```python
from build123d import *

# Parameters (mm, degrees)
SKETCH_1_R          = 2
EXTRUDE_1_DEPTH     = 5
SKETCH_2_R          = 0.35
SKETCH_5_R          = 2.75
SKETCH_5_R_2        = 1.75
CUT_EXTRUDE_1_DEPTH = 4


with BuildPart() as part:
    # Эскиз1 → Бобышка-Вытянуть1 (new body)
    with BuildSketch(Plane(origin=(0, 0, 0), x_dir=(0, 0, -1), z_dir=(1, 0, 0))):
        Circle(SKETCH_1_R)
    extrude_1 = extrude(amount=EXTRUDE_1_DEPTH)

    # По траектории1: sweep along a path in Эскиз3
    with BuildLine(Plane.XY) as sweep_1_path:
        Line((5, 0), (9.16, 0))
        ThreePointArc((9.16, 0), (9.867106781, -0.292893219), (10.16, -1))
        Line((10.16, -1), (10.16, -8))
    # Эскиз2 → По траектории1 (sweep)
    with BuildSketch(Plane(origin=(5, 0, 0), x_dir=(0, 0, -1), z_dir=(1, 0, 0))):
        Circle(SKETCH_2_R)
    sweep_1 = sweep(path=sweep_1_path.line)

    # Зеркальное отражение1: Бобышка-Вытянуть1, По траектории1 across Right Plane
    add(extrude_1.mirror(Plane(origin=(0, 0, 0), x_dir=(0, 0, -1), z_dir=(1, 0, 0))))
    add(sweep_1.mirror(Plane(origin=(0, 0, 0), x_dir=(0, 0, -1), z_dir=(1, 0, 0))))

    # Эскиз5 → Вырез-Вытянуть-Тонкостенный1 (cut, symmetric)
    with BuildSketch(Plane(origin=(0, 0, 0), x_dir=(0, 0, -1), z_dir=(1, 0, 0))):
        Circle(SKETCH_5_R)
        Circle(SKETCH_5_R_2, mode=Mode.SUBTRACT)
    extrude(amount=CUT_EXTRUDE_1_DEPTH, both=True, mode=Mode.SUBTRACT)


solid = part.part
```
Verification items for the finished model (mm, model axes). Round coordinates to 2 decimals unless told otherwise and drop trailing zeros. Write each loop counter-clockwise with the first axis right and the second up, starting at its lowest first coordinate (ties: lowest second). Pieces come first, ordered by that corner, then holes. Notation, with made-up numbers: (68.5, 87) - (92.5, 87) arc R27 cw to (92.5, 124) - close; hole circle Ø8 at (9, 11.25). An arc over 180 degrees is marked (long way). Answer as a JSON object with one key per item and string values. Group by question number.
Q1. Thickness scan on line 1 (X direction, y = 1.75, z = 0.65); line 2 (X direction, y = 0.5, z = -1.6); line 3 (Y direction, x = -0.5, z = -0.1). Record the ranges inside material, lowest first.
Q2. Section check C-C, the plane x = 6. Enter the section's corners in (y, z), plus the area to 3 significant figures.
Q3. Section check B-B, the plane y = -7. Enter the section's corners in (x, z), plus the area to 3 significant figures.
Q4. Go/stop test with flat-tipped pins: pin 1 Ø1.2 at (y, z) = (1, 0.5) entering from -X; pin 2 Ø1.5 at (x, z) = (8, 0.5) entering from +Y; pin 3 Ø2 at (y, z) = (-0.5, 0) entering from +X; pin 4 Ø2 at (y, z) = (0.5, -0.5) entering from +X. Record where each tip stops, or that it passes through.
Q5. Section check D-D, the plane z = 1.2. Enter the section's corners in (x, y), plus the area to 3 significant figures.
Q6. Section check A-A, the plane z = 0. Enter the section's corners in (x, y).
Found:
{
 "1": {"line 1": "x = -5 to -4, 4 to 5", "line 2": "x = -5 to 5", "line 3": "y = -1.75 to 1.75"},
 "2": {"outline": "circle Ø0.7 at (0, 0)", "area": "0.385 mm^2"},
 "3": {"outline": "circle Ø0.7 at (-10.16, 0); circle Ø0.7 at (10.16, 0)", "area": "0.770 mm^2"},
 "4": {"pin 1": "stops at x = -5", "pin 2": "stops at y = 0.35", "pin 3": "stops at x = 10.51", "pin 4": "stops at x = 10.36"},
 "5": {"outline": "(-5, -1.6) - (-4, -1.6) - (-4, -1.27) - (4, -1.27) - (4, -1.6) - (5, -1.6) - (5, 1.6) - (4, 1.6) - (4, 1.27) - (-4, 1.27) - (-4, 1.6) - (-5, 1.6) - close", "area": "26.8 mm^2"},
 "6": {"outline": "(-10.51, -8) - (-9.81, -8) - (-9.81, -1) arc R0.65 cw to (-9.16, -0.35) - (-5, -0.35) - (-5, -2) - (-4, -2) - (-4, -1.75) - (4, -1.75) - (4, -2) - (5, -2) - (5, -0.35) - (9.16, -0.35) arc R0.65 cw to (9.81, -1) - (9.81, -8) - (10.51, -8) - (10.51, -1) arc R1.35 ccw to (9.16, 0.35) - (5, 0.35) - (5, 2) - (4, 2) - (4, 1.75) - (-4, 1.75) - (-4, 2) - (-5, 2) - (-5, 0.35) - (-9.16, 0.35) arc R1.35 ccw to (-10.51, -1) - close"}
}
